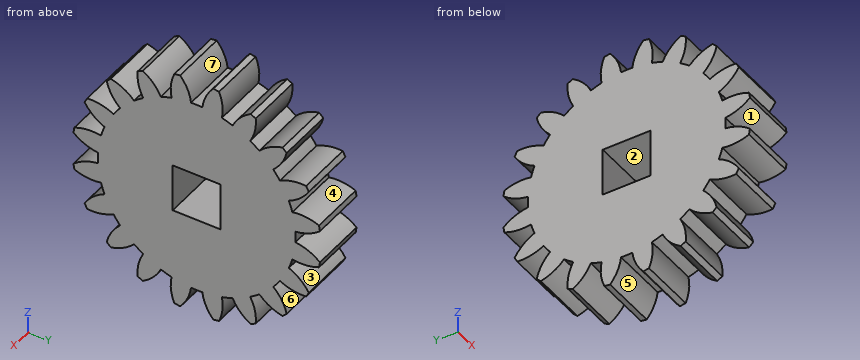
```python
from build123d import *

# Parameters (mm, degrees)
BASPROSKE_W        = 5
BASPROSKE_H        = 11
TOOTHCUT_DEPTH     = 17.340134638
TEETHCUTS_COUNT    = 20
TEETHCUTS_ANGLE    = 342
BORSKE_R           = 0.4
BORE_DEPTH         = 50.0000508
SKETCH1_W          = 4.242640688
SKETCH1_H          = 4.242640688
CUT_EXTRUDE1_DEPTH = 17.208263488


with BuildPart() as part:
    # BasProSke → Base-Revolve (revolve)
    with BuildSketch(Plane(origin=(0, 0, 0), x_dir=(1, 0, 0), z_dir=(0, 1, 0)), mode=Mode.PRIVATE) as base_revolve_sk:
        with Locations((2.5, 5.5)):
            Rectangle(BASPROSKE_W, BASPROSKE_H)
    revolve(base_revolve_sk.sketch.rotate(Axis((-10, 0, 0), (1, 0, 0)), 180), axis=Axis((-10, 0, 0), (1, 0, 0)))

    # TooCutSke → ToothCut (cut, through all)
    with BuildSketch(Plane(origin=(0, 0, 0), x_dir=(0, 0, -1), z_dir=(1, 0, 0))):
        with BuildLine():
            ThreePointArc((0.499924007, 8.734705318), (0, 8.749), (-0.499924007, 8.734705318))
            ThreePointArc((-0.499924007, 8.734705318), (-0.824302243, 9.905497836), (-1.485192705, 10.924909509))
            ThreePointArc((-1.485192705, 10.924909509), (0, 11.0254), (1.485192705, 10.924909509))
            ThreePointArc((1.485192705, 10.924909509), (0.824302243, 9.905497836), (0.499924007, 8.734705318))
        make_face()
    toothcut = extrude(amount=TOOTHCUT_DEPTH, mode=Mode.SUBTRACT)

    # TeethCuts: ToothCut ×20 about axis
    teethcuts_axis = Axis((-10, 0, 0), (1, 0, 0))
    for i in range(1, TEETHCUTS_COUNT):
        add(toothcut.rotate(teethcuts_axis, i * TEETHCUTS_ANGLE / (TEETHCUTS_COUNT - 1)), mode=Mode.SUBTRACT)

    # BorSke → Bore (cut, symmetric)
    with BuildSketch(Plane(origin=(0, 0, 0), x_dir=(0, 0, -1), z_dir=(1, 0, 0))):
        with Locations(Location((0, 0, 0), (0, 0, 180))):
            Circle(BORSKE_R)
    extrude(amount=BORE_DEPTH, both=True, mode=Mode.SUBTRACT)

    # Sketch1 → Cut-Extrude1 (cut, through all)
    with BuildSketch(Plane(origin=(5, 0, 0), x_dir=(0, 0, -1), z_dir=(1, 0, 0))):
        Rectangle(SKETCH1_W, SKETCH1_H)
    extrude(amount=-CUT_EXTRUDE1_DEPTH, mode=Mode.SUBTRACT)


solid = part.part
```
Check sheet for the modelled part. Datum: model origin and axes. Units: mm. Face numbers are marked on the shaded views. A direction names the side the tool comes from. Give positions to 0.01 mm unless a question says otherwise; leave off trailing zeros. Write each loop counter-clockwise with the first axis right and the second up, starting at its lowest first coordinate (ties: lowest second). Pieces come first, ordered by that corner, then holes. Notation, with made-up numbers: (-20.5, 7.25) - (2.5, 7.25) arc R19 cw to (2.5, 29.25) - close; hole circle Ø1 at (-28, 38.25). An arc over 180 degrees is marked (long way). Answer as a JSON object with one key per item and string values. Group by question number.
1) Access from +Z, -Z, +X, -X, +Y, -Y to the whole of each face (thin tool, end or side, straight path). Record for the marked faces 4, 5, 6 and 7.
2) Thickness scan on probe 1 along Y at (x, z) = (3.55, -0.25); probe 2 along Z at (x, y) = (3.4, -7). Record the ranges inside material, lowest first. Write a range as from..to.
3) Sectioned sample at A-A (z = -4.25). Record the cut outline in (x, y).
4) Sectioned sample at B-B (y = -3.75). Record the cut outline in (x, z), then the cut area to 3 significant figures.
5) Release check for a two-part mould opening along Y. For the marked faces 1, 2 and 3 record: pulls with the +Y half, pulls with the -Y half, needs draft (parallel to the pull), parting line crosses it, or undercut.
6) Depth check by flat-ended pin: P1, Ø2, axis at y = -8.5, z = -8, coming from the +X side; P2, Ø1, axis at x = 1, z = -8, coming from the -Y side. Enter the tip coordinate at first touch or a pass-through.
Geometry results:
{
 "1": {"face 4": "+X, -X", "face 5": "-Z, +X, -X", "face 6": "+X, -X, +Y", "face 7": "+Z, +X, -X"},
 "2": {"probe 1": "y = -8.75..-2.12, 2.12..8.75", "probe 2": "z = -7.78..-5.77, -5.25..5.25, 5.77..7.78"},
 "3": {"outline": "(0, -9.55) - (5, -9.55) - (5, 9.55) - (0, 9.55) - close"},
 "4": {"outline": "(0, -9.06) - (5, -9.06) - (5, 9.06) - (0, 9.06) - close", "area": "90.6 mm^2"},
 "5": {"face 1": "pulls with the -Y half", "face 2": "undercut", "face 3": "pulls with the +Y half"},
 "6": {"P1": "stops at x = 5", "P2": "stops at y = -7.96"}
}
